Geometry: final body of the model. Coordinates: model frame, mm. Face numbers are marked on the shaded views. A direction names the side the tool comes from. Round coordinates to 2 decimals unless told otherwise and drop trailing zeros. Write each loop counter-clockwise with the first axis right and the second up, starting at its lowest first coordinate (ties: lowest second). Pieces come first, ordered by that corner, then holes. Notation, with made-up numbers: (21, 6) -> (35, 6) arc R23 cw to (35, 27) -> close; hole circle Ø7 at (-38.75, 25). An arc over 180 degrees is marked (long way). Use one line per item in the form item = value. Start each with the question number.
1. Reachability of the marked faces 1 and 2 from +Z, -Z, +X, -X, +Y, -Y: full face, straight path, thin tool, end or side. Return the list, or none.
2. Cut plane D-D, the plane x = 12.7. Return the cut outline in (y, z).
3. Cut plane B-B, the plane y = 51.75. Return the cut outline in (x, z), plus the area to 3 significant figures.
4. Pin query (flat end, axial travel): pin 1 Ø2 at (x, y) = (31, 27.5) entering from -Z; pin 2 Ø4 at (x, z) = (53.98, -48.04) entering from -Y; pin 3 Ø10 at (x, z) = (-20.64, -21.05) entering from +Y. Return the tip coordinate at first contact, or that it passes through.
5. Line query: L1, parallel to Z at x = 4.5, y = 37; L2, parallel to Y at x = 12, z = -1; L3, parallel to Y at x = -13.5, z = -7.5. Output: solid intervals per line, ascending.
6. Cut plane C-C, the plane z = -33.75. Return the cut outline in (x, y) (1 decimal), plus the area to 4 significant figures.
7. Cut plane A-A, the plane x = 68.6. Return the cut outline in (y, z).
```python
from build123d import *

# Parameters (mm, degrees)
SKETCH1_R           = 3.175
SKETCH1_R_2         = 1.5
BOSS_EXTRUDE1_DEPTH = 2
BOSS_EXTRUDE2_DEPTH = 50.8
SKETCH3_R           = 1.7
SKETCH3_R_2         = 3.175
CUT_EXTRUDE1_DEPTH  = 120.575917308


with BuildPart() as part:
    # Sketch1 → Boss-Extrude1 (new body)
    with BuildSketch(Plane.XY):
        Polygon((0, 58.4), (60.325, 58.4), (60.325, 71.1), (90, 71.1), (90, 0), (0, 0), align=None)
        with Locations((68.6, 56.33204182)):
            Circle(SKETCH1_R, mode=Mode.SUBTRACT)
        with Locations((12.7, 51.75)):
            Circle(SKETCH1_R_2, mode=Mode.SUBTRACT)
        with Locations((38.1, 51.75)):
            Circle(SKETCH1_R_2, mode=Mode.SUBTRACT)
        with Locations((12.7, 4.65)):
            Circle(SKETCH1_R_2, mode=Mode.SUBTRACT)
        with Locations((38.1, 4.65)):
            Circle(SKETCH1_R_2, mode=Mode.SUBTRACT)
    extrude(amount=-BOSS_EXTRUDE1_DEPTH)

    # Sketch2 → Boss-Extrude2 (add)
    with BuildSketch(Plane(origin=(0, 0, -2), x_dir=(-1, 0, 0), z_dir=(0, 0, -1))):
        Polygon((0, 56.4), (41.275, 56.4), (41.275, 58.4), (0, 58.4), (-60.325, 58.4), (-60.325, 56.4), align=None)
    extrude(amount=BOSS_EXTRUDE2_DEPTH)

    # Sketch3 → Cut-Extrude1 (cut, through all)
    with BuildSketch(Plane(origin=(0, 58.4, 0), x_dir=(1, 0, 0), z_dir=(0, 1, 0))):
        with Locations(Location((53.975, 48.0375, 0), (0, 0, 270))):
            Circle(SKETCH3_R)
        with Locations(Location((53.975, 6.7625, 0), (0, 0, 270))):
            Circle(SKETCH3_R)
        with Locations(Location((-20.6375, 33.75, 0), (0, 0, 270))):
            Circle(SKETCH3_R_2)
        with Locations(Location((-20.6375, 21.05, 0), (0, 0, 270))):
            Circle(SKETCH3_R_2)
    extrude(amount=-CUT_EXTRUDE1_DEPTH, mode=Mode.SUBTRACT)


solid = part.part
```
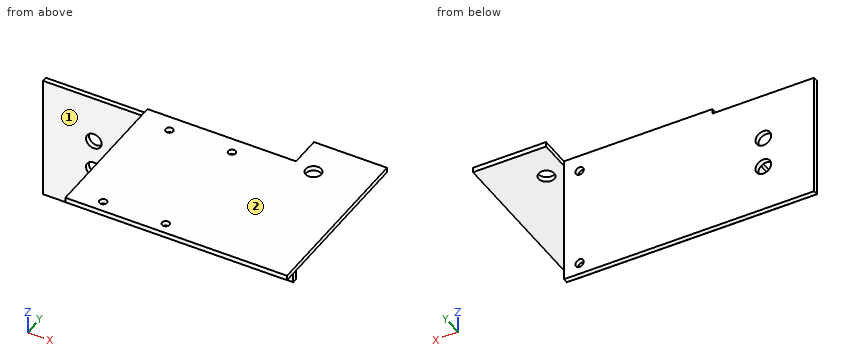
Outcome:
q1.face_1 = -Z, +X, -X, -Y
q1.face_2 = +Z, +X, -X, +Y, -Y
q2.outline = (0, -2) -> (3.15, -2) -> (3.15, 0) -> (0, 0) -> close; (6.15, -2) -> (50.25, -2) -> (50.25, 0) -> (6.15, 0) -> close; (53.25, -2) -> (56.4, -2) -> (56.4, -52.8) -> (58.4, -52.8) -> (58.4, 0) -> (53.25, 0) -> close
q3.outline = (0, -2) -> (11.2, -2) -> (11.2, 0) -> (0, 0) -> close; (14.2, -2) -> (36.6, -2) -> (36.6, 0) -> (14.2, 0) -> close; (39.6, -2) -> (90, -2) -> (90, 0) -> (39.6, 0) -> close
q3.area = 168 mm^2
q4.pin_1 = -2
q4.pin_2 = 56.4
q4.pin_3 = 58.4
q5.L1 = -2 to 0
q5.L2 = 0 to 3.32, 5.98 to 50.42, 53.08 to 58.4
q5.L3 = 56.4 to 58.4
q6.outline = (-41.3, 56.4) -> (-23.8, 56.4) -> (-23.8, 58.4) -> (-41.3, 58.4) -> close; (-17.5, 56.4) -> (60.3, 56.4) -> (60.3, 58.4) -> (-17.5, 58.4) -> close
q6.area = 190.5 mm^2
q7.outline = (0, -2) -> (53.16, -2) -> (53.16, 0) -> (0, 0) -> close; (59.51, -2) -> (71.1, -2) -> (71.1, 0) -> (59.51, 0) -> close
